from build123d import *

# Parameters (mm, degrees)
SKETCH_2_R                   = 6
EXTRUDE_1_DEPTH              = 16.5
SKETCH_3_R                   = 3.25
CUT_EXTRUDE_1_DEPTH          = 13
CUT_EXTRUDE_START            = -13
SKETCH_4_R                   = 3.25
CUT_EXTRUDE_2_DEPTH          = 13
EXTRUDE_2_DEPTH              = 16.5
CUT_EXTRUDE_4_DEPTH          = 1.95
CUT_EXTRUDE_4_DEPTH_BACK     = 1.95
CUT_EXTRUDE_5_DEPTH          = 1.95
CUT_EXTRUDE_5_DEPTH_BACK     = 1.95
PATTERN_CIRCULAR_1_COUNT     = 3
EXTRUDE_3_DEPTH              = 3.5
CUT_EXTRUDE_3_DEPTH          = 54.725986169
CUT_EXTRUDE_3_DEPTH_BACK     = 54.725986169
SKETCH_9_R                   = 3
HOLE_WIZARD_M4_1_D           = 4.5
HOLE_WIZARD_M4_1_CBORE_D     = 9
HOLE_WIZARD_M4_1_CBORE_DEPTH = 2


with BuildPart() as part:
    # Sketch 2 → Extrude 1 (new, symmetric)
    with BuildSketch(Plane(origin=(0, 0, 0), x_dir=(0, 0, -1), z_dir=(1, 0, 0))):
        with Locations((0, -30)):
            Circle(SKETCH_2_R)
    extrude(amount=EXTRUDE_1_DEPTH, both=True)

    # Sketch 3 → Cut-Extrude 1 (cut)
    with BuildSketch(Plane(origin=(16.5, 0, 0), x_dir=(0, 0, -1), z_dir=(1, 0, 0))):
        with Locations((0, -30)):
            Circle(SKETCH_3_R)
    extrude(amount=-CUT_EXTRUDE_1_DEPTH, mode=Mode.SUBTRACT)

    # Sketch 4 → Cut-Extrude 2 (cut)
    with BuildSketch(Plane.ZY.offset(16.5).offset(CUT_EXTRUDE_START)):
        with Locations(Location((0, -30, 0), (0, 0, 180))):
            Circle(SKETCH_4_R)
    extrude(amount=CUT_EXTRUDE_2_DEPTH, mode=Mode.SUBTRACT)

    # Sketch 6 → Extrude 2 (add, symmetric)
    with BuildSketch(Plane(origin=(0, 0, 0), x_dir=(0, 0, -1), z_dir=(1, 0, 0))):
        with BuildLine():
            Line((-3.5, -23.876275643), (-3.5, -22))
            Line((-3.5, -22), (3.5, -22))
            Line((3.5, -22), (3.5, -23.876275643))
            ThreePointArc((3.5, -23.876275643), (3.703994726, -24.915677944), (4.285714286, -25.800874727))
            Line((4.285714286, -25.800874727), (-4.285714286, -25.800874727))
            ThreePointArc((-4.285714286, -25.800874727), (-3.703994726, -24.915677944), (-3.5, -23.876275643))
        make_face()
    extrude(amount=EXTRUDE_2_DEPTH, both=True)

    # Sketch 12 → Cut-Extrude 4 (cut, two sides: drawn at the far end of the back side and taken through both)
    with BuildSketch(Plane.ZY.offset(10.5).offset(-CUT_EXTRUDE_4_DEPTH_BACK)):
        Polygon((-4.2, -36), (4.2, -36), (4.2, -32.424871131), (0, -34.849742261), (-4.2, -32.424871131), align=None)
        Polygon((-4.2, -27.575128869), (-4.2, -32.424871131), (0, -34.849742261), (4.2, -32.424871131), (4.2, -27.575128869), (0, -25.150257739), align=None)
    extrude(amount=CUT_EXTRUDE_4_DEPTH + CUT_EXTRUDE_4_DEPTH_BACK, mode=Mode.SUBTRACT)

    # Sketch 13 → Cut-Extrude 5 (cut, two sides: drawn at the far end of the back side and taken through both)
    with BuildSketch(Plane(origin=(10.5, 0, 0), x_dir=(0, 0, -1), z_dir=(1, 0, 0)).offset(-CUT_EXTRUDE_5_DEPTH_BACK)):
        with BuildLine():
            Line((-4.2, -27.575128869), (-4.2, -34.284857057))
            ThreePointArc((-4.2, -34.284857057), (0, -36), (4.2, -34.284857057))
            Line((4.2, -34.284857057), (4.2, -27.575128869))
            Line((4.2, -27.575128869), (0, -25.150257739))
            Line((0, -25.150257739), (-4.2, -27.575128869))
        make_face()
    extrude(amount=CUT_EXTRUDE_5_DEPTH + CUT_EXTRUDE_5_DEPTH_BACK, mode=Mode.SUBTRACT)


with BuildPart() as pattern_circular_1_1:
    # Pattern Circular 1: pattern copy
    add(part.part.rotate(Axis((0, 0, 0), (0, 0, 1)), 1 * 360 / PATTERN_CIRCULAR_1_COUNT))


with BuildPart() as pattern_circular_1_2:
    # Pattern Circular 1: pattern copy
    add(part.part.rotate(Axis((0, 0, 0), (0, 0, 1)), 2 * 360 / PATTERN_CIRCULAR_1_COUNT))


with BuildPart() as part_1:
    add(part.part)

    add(pattern_circular_1_1.part)  # Extrude 3 merges Pattern Circular 1_1

    add(pattern_circular_1_2.part)  # Extrude 3 merges Pattern Circular 1_2
    # Sketch 8 → Extrude 3 (add, symmetric)
    with BuildSketch(Plane.XY):
        with BuildLine():
            Line((16.5, -22), (-16.5, -22))
            Line((-16.5, -22), (-16.5, -17.434263876))
            ThreePointArc((-16.5, -17.434263876), (-16.548246013, -17.067799022), (-16.689696167, -16.726308143))
            Line((-16.689696167, -16.726308143), (-22.830255847, -6.090546791))
            ThreePointArc((-22.830255847, -6.090546791), (-23.055270547, -5.797301924), (-23.348515413, -5.572287224))
            Line((-23.348515413, -5.572287224), (-27.302558883, -3.289419162))
            Line((-27.302558883, -3.289419162), (-10.802558883, 25.289419162))
            Line((-10.802558883, 25.289419162), (-6.848515413, 23.0065511))
            ThreePointArc((-6.848515413, 23.0065511), (-6.507024533, 22.865100947), (-6.14055968, 22.816854933))
            Line((-6.14055968, 22.816854933), (6.14055968, 22.816854933))
            ThreePointArc((6.14055968, 22.816854933), (6.507024533, 22.865100947), (6.848515413, 23.0065511))
            Line((6.848515413, 23.0065511), (10.802558883, 25.289419162))
            Line((10.802558883, 25.289419162), (27.302558883, -3.289419162))
            Line((27.302558883, -3.289419162), (23.348515413, -5.572287224))
            ThreePointArc((23.348515413, -5.572287224), (23.055270547, -5.797301924), (22.830255847, -6.090546791))
            Line((22.830255847, -6.090546791), (16.689696167, -16.726308143))
            ThreePointArc((16.689696167, -16.726308143), (16.548246013, -17.067799022), (16.5, -17.434263876))
            Line((16.5, -17.434263876), (16.5, -22))
        make_face()
    extrude(amount=EXTRUDE_3_DEPTH, both=True)

    # Sketch 9 → Cut-Extrude 3 (cut, two sides: drawn at the far end of the back side and taken through both)
    with BuildSketch(Plane.XY.offset(-CUT_EXTRUDE_3_DEPTH_BACK)):
        Circle(SKETCH_9_R)
    extrude(amount=CUT_EXTRUDE_3_DEPTH + CUT_EXTRUDE_3_DEPTH_BACK, mode=Mode.SUBTRACT)

    # Hole Wizard M4 _ _ _ _1 (through all)
    with Locations(Plane.XY.offset(3.5)):
        with Locations((0, 9), (7.794228634, -4.5), (-7.794228634, -4.5)):
            CounterBoreHole(HOLE_WIZARD_M4_1_D / 2, HOLE_WIZARD_M4_1_CBORE_D / 2, HOLE_WIZARD_M4_1_CBORE_DEPTH)


solid = part_1.part
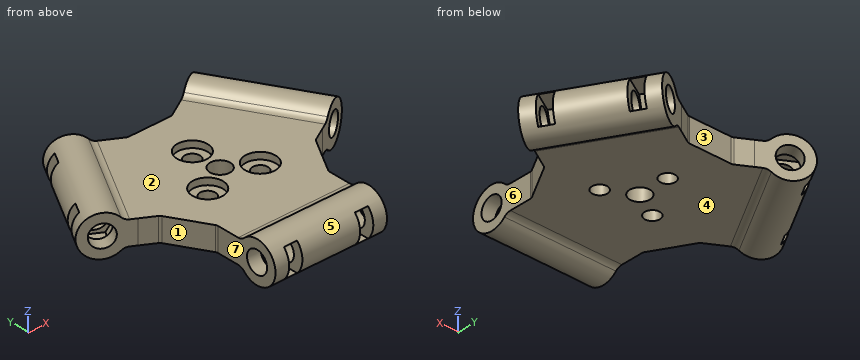
Check sheet for the modelled part. Datum: model origin and axes. Units: mm. Face numbers are marked on the shaded views. A direction names the side the tool comes from. Coordinates: 2 decimals unless noted, no trailing zeros. Write each loop counter-clockwise with the first axis right and the second up, starting at its lowest first coordinate (ties: lowest second). Pieces come first, ordered by that corner, then holes.
Item 1: Scan lines: probe 1 along Z at (x, y) = (-5, -30); probe 2 along Y at (x, z) = (0, 2.1); probe 3 along Y at (x, z) = (15.35, 0). Record each from-to range of solid material in increasing order.
Numbers:
probe 1: z = -6 to -3.25, 3.25 to 6
probe 2: y = -35.62 to -3, 3 to 4.5, 13.5 to 22.82
probe 3: y = -36 to -33.25, -26.75 to 26.91
Item 2: Cross-section at A-A on x = 0. Record the boundary of the cut face in (y, z), then the cut area to 3 significant figures.
Numbers:
outline: (-25.8, -4.29) arc R2.75 cw to (-23.88, -3.5) - (-3, -3.5) - (-3, 3.5) - (-23.88, 3.5) arc R2.75 cw to (-25.8, 4.29) arc R6 ccw (long way) to start; (3, -3.5) - (6.75, -3.5) - (6.75, 1.5) - (4.5, 1.5) - (4.5, 3.5) - (3, 3.5) - close; (11.25, -3.5) - (22.82, -3.5) - (22.82, 3.5) - (13.5, 3.5) - (13.5, 1.5) - (11.25, 1.5) - close
area: 361 mm2
Item 3: Cross-section at D-D on y = -30. Record the boundary of the cut face in (x, z), then the cut area to 3 significant figures.
Numbers:
outline: (-16.5, -6) - (16.5, -6) - (16.5, -3.25) - (12.45, -3.25) - (12.45, -4.2) - (8.55, -4.2) - (8.55, -3.25) - (3.5, -3.25) - (3.5, 3.25) - (8.55, 3.25) - (8.55, 4.2) - (12.45, 4.2) - (12.45, 3.25) - (16.5, 3.25) - (16.5, 6) - (-16.5, 6) - (-16.5, 3.25) - (-12.45, 3.25) - (-12.45, 4.2) - (-8.55, 4.2) - (-8.55, 3.25) - (-3.5, 3.25) - (-3.5, -3.25) - (-8.55, -3.25) - (-8.55, -4.2) - (-12.45, -4.2) - (-12.45, -3.25) - (-16.5, -3.25) - close
area: 212 mm2
Item 4: Cross-section at B-B on y = -4.5. Record the boundary of the cut face in (x, z).
Numbers:
outline: (-25.21, -3.5) - (-10.04, -3.5) - (-10.04, 1.5) - (-12.29, 1.5) - (-12.29, 3.5) - (-25.21, 3.5) - close; (-5.54, -3.5) - (5.54, -3.5) - (5.54, 1.5) - (3.29, 1.5) - (3.29, 3.5) - (-3.29, 3.5) - (-3.29, 1.5) - (-5.54, 1.5) - close; (10.04, -3.5) - (25.21, -3.5) - (25.21, 3.5) - (12.29, 3.5) - (12.29, 1.5) - (10.04, 1.5) - close
Item 5: Access from +Z, -Z, +X, -X, +Y, -Y to the whole of each face (thin tool, end or side, straight path). Record for the marked faces 5, 6 and 7.
Numbers:
face 5: +X, -X
face 6: +Z, -Z, +X, -Y
face 7: +Z, -Z, -X, -Y
Item 6: Depth check by flat-ended pin: pin 1 Ø1.5 at (x, z) = (18, 0.5) entering from +Y; pin 2 Ø6 at (y, z) = (-17.5, 2.5) entering from +X; pin 3 Ø25 at (x, y) = (9.5, 5.5) entering from +Z. Enter the tip coordinate at first touch or a pass-through.
Numbers:
pin 1: stops at y = 21.26
pin 2: stops at x = 17.98
pin 3: stops at z = 3.5
Item 7: Cross-section at C-C on z = -1.5. Count the separate pieces of the cut face and the enclosed holes in it, then the cut area to 3 significant figures.
Numbers:
separate pieces: 7
enclosed holes: 4
area: 2,530 mm2
Item 8: Mould release check, pull along Y, two halves, no side actions. Record for the marked faces 1, 2, 3 and 4: released by +Y, released by -Y, zero draft, split by the parting line, or undercut.
Numbers:
face 1: released by -Y
face 2: undercut
face 3: released by +Y
face 4: undercut
